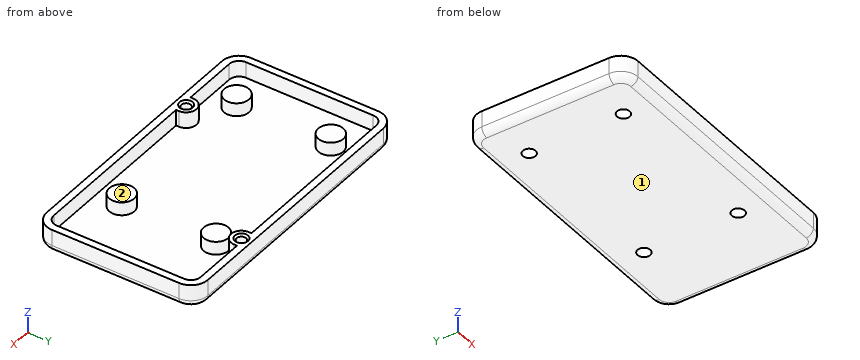
from build123d import *

# Parameters (mm, degrees)
PAD_DEPTH         = 3.4
THICKNESS_T       = 1.5
CYLINDER_W        = 2.2
CYLINDER_H        = 3.4
CYLINDER_ANGLE    = 180
BOX004_W          = 4.4
BOX004_H          = 0.6
BOX004_DEPTH      = 3.4
CYLINDER002_R     = 1
CYLINDER002_DEPTH = 3.9
CHAMFER_SIZE      = 0.4
CYLINDER003_W     = 2.2
CYLINDER003_H     = 3.4
CYLINDER003_ANGLE = 180
BOX006_W          = 4.4
BOX006_H          = 0.6
BOX006_DEPTH      = 3.4
CYLINDER004_R     = 1
CYLINDER004_DEPTH = 3.9
CHAMFER001_SIZE   = 0.4
SKETCH004_R       = 2.65
PAD002_DEPTH      = 2.8
SKETCH005_R       = 1.35
POCKET001_DEPTH   = 3.5


with BuildPart() as part:
    # Sketch → Pad (new body)
    with BuildSketch(Plane.XY):
        with BuildLine():
            Line((2, 31.1), (55.5, 31.1))
            ThreePointArc((57.6, 29), (56.984924, 30.484924), (55.5, 31.1))
            Line((57.6, 29), (57.6, 2))
            ThreePointArc((55.5, -0.1), (56.984924, 0.515076), (57.6, 2))
            Line((55.5, -0.1), (2, -0.1))
            ThreePointArc((-0.1, 2), (0.515076, 0.515076), (2, -0.1))
            Line((-0.1, 2), (-0.1, 29))
            ThreePointArc((2, 31.1), (0.515076, 30.484924), (-0.1, 29))
        make_face()
    extrude(amount=-PAD_DEPTH)

    # Thickness
    thickness_openings = [part.faces().sort_by_distance(p)[0] for p in [
        (28.75, 15.5, 0),
    ]]
    offset(amount=THICKNESS_T, openings=thickness_openings)

    # Cylinder → Cylinder (revolve)
    with BuildSketch(Plane(origin=(16, 0.5, -3.4), x_dir=(1, 0, 0), z_dir=(0, -1, 0))):
        with Locations((1.1, 1.7)):
            Rectangle(CYLINDER_W, CYLINDER_H)
    revolve(axis=Axis((16, 0.5, -3.4), (0, 0, 1)), revolution_arc=CYLINDER_ANGLE)

    # Box004 → Box004 (join)
    with BuildSketch(Plane(origin=(13.8, -0.1, -3.4), x_dir=(1, 0, 0), z_dir=(0, 0, 1))):
        with Locations((2.2, 0.3)):
            Rectangle(BOX004_W, BOX004_H)
    extrude(amount=BOX004_DEPTH)

    # Cylinder002 → Cylinder002 (cut)
    with BuildSketch(Plane(origin=(16, 0.5, -3.9), x_dir=(1, 0, 0), z_dir=(0, 0, 1))):
        Circle(CYLINDER002_R)
    extrude(amount=CYLINDER002_DEPTH, mode=Mode.SUBTRACT)

    # Chamfer
    chamfer_edges = [part.edges().sort_by_distance(p)[0] for p in [
        (16, 1.5, 0),
        (16, -0.5, 0),
        (15.051317, 0.183772, 0),
        (16.948683, 0.183772, 0),
    ]]
    chamfer(chamfer_edges, length=CHAMFER_SIZE)

    # Cylinder003 → Cylinder003 (revolve)
    with BuildSketch(Plane(origin=(42.25, 30.5, -3.4), x_dir=(-1, 0, 0), z_dir=(0, 1, 0))):
        with Locations((1.1, 1.7)):
            Rectangle(CYLINDER003_W, CYLINDER003_H)
    revolve(axis=Axis((42.25, 30.5, -3.4), (0, 0, 1)), revolution_arc=CYLINDER003_ANGLE)

    # Box006 → Box006 (join)
    with BuildSketch(Plane(origin=(40.05, 30.5, -3.4), x_dir=(1, 0, 0), z_dir=(0, 0, 1))):
        with Locations((2.2, 0.3)):
            Rectangle(BOX006_W, BOX006_H)
    extrude(amount=BOX006_DEPTH)

    # Cylinder004 → Cylinder004 (cut)
    with BuildSketch(Plane(origin=(42.25, 30.5, -3.9), x_dir=(1, 0, 0), z_dir=(0, 0, 1))):
        Circle(CYLINDER004_R)
    extrude(amount=CYLINDER004_DEPTH, mode=Mode.SUBTRACT)

    # Chamfer001
    chamfer001_edges = [part.edges().sort_by_distance(p)[0] for p in [
        (42.25, 31.5, 0),
        (43.198683, 30.816228, 0),
        (42.25, 29.5, 0),
        (41.301317, 30.816228, 0),
    ]]
    chamfer(chamfer001_edges, length=CHAMFER001_SIZE)

    # Sketch004 → Pad002 (join)
    with BuildSketch(Plane.XY.offset(-3.4)):
        with Locations((7.8, 5.5)):
            Circle(SKETCH004_R)
        with Locations((42.8, 5.5)):
            Circle(SKETCH004_R)
        with Locations((7.8, 25.5)):
            Circle(SKETCH004_R)
        with Locations((42.8, 25.5)):
            Circle(SKETCH004_R)
    extrude(amount=PAD002_DEPTH)

    # Sketch005 → Pocket001 (cut)
    with BuildSketch(Plane.XY.offset(-4.9)):
        with Locations((7.8, 5.5)):
            Circle(SKETCH005_R)
        with Locations((42.8, 5.5)):
            Circle(SKETCH005_R)
        with Locations((7.8, 25.5)):
            Circle(SKETCH005_R)
        with Locations((42.8, 25.5)):
            Circle(SKETCH005_R)
    extrude(amount=POCKET001_DEPTH, mode=Mode.SUBTRACT)


solid = part.part
Part model, mm, in its own coordinate system. Face numbers are marked on the shaded views. Round coordinates to 2 decimals unless told otherwise and drop trailing zeros. Write each loop counter-clockwise with the first axis right and the second up, starting at its lowest first coordinate (ties: lowest second). Pieces come first, ordered by that corner, then holes. Notation, with made-up numbers: M 63,-3.5 L 88,-3.5 A11 cw 88,15.5 Z; hole C -20.75,8 d11. An arc over 180 degrees is marked long. Return JSON: item names as keys, results as strings. Group by question number.
(1) Saw through at B-B on x = 7.8. Write the cut outline in (y, z).
(2) Saw through at C-C on y = 5.5. Write the cut outline in (x, z).
(3) Two-plate mould, pull along Y, no slides. Class the marked faces 1 and 2: +Y half, -Y half, draft (parallel to the pull), parting line (faces both ways), or undercut.
(4) Saw through at D-D on x = 20.5. Write the cut outline in (y, z), then the cut area to 3 significant figures.
(5) Pin check, flat tips, straight feed: pin 1 Ø2 at (x, y) = (43, 25.5) entering from -Z; pin 2 Ø4.5 at (x, y) = (42.8, 25.5) entering from +Z; pin 3 Ø0.7 at (y, z) = (0, -2) entering from +X. Stop position of each tip, or through.
(6) Drill centre lines: probe 1 along Y at (x, z) = (55.5, -0.65); probe 2 along Y at (x, z) = (16, -2.95); probe 3 along Y at (x, z) = (42, -4.5). Where is each one in solid material? Low to high.
(7) Saw through at A-A on y = 19. Write the cut outline in (x, z), then the cut area to 3 significant figures.
Returned:
{
 "1": {"outline": "M -1.6,-3.4 A1.5 ccw -0.1,-4.9 L 4.15,-4.9 L 4.15,-1.4 L 6.85,-1.4 L 6.85,-4.9 L 24.15,-4.9 L 24.15,-1.4 L 26.85,-1.4 L 26.85,-4.9 L 31.1,-4.9 A1.5 ccw 32.6,-3.4 L 32.6,0 L 31.1,0 L 31.1,-3.4 L 28.15,-3.4 L 28.15,-0.6 L 22.85,-0.6 L 22.85,-3.4 L 8.15,-3.4 L 8.15,-0.6 L 2.85,-0.6 L 2.85,-3.4 L -0.1,-3.4 L -0.1,0 L -1.6,0 Z"},
 "2": {"outline": "M -1.6,-3.4 A1.5 ccw -0.1,-4.9 L 6.45,-4.9 L 6.45,-1.4 L 9.15,-1.4 L 9.15,-4.9 L 41.45,-4.9 L 41.45,-1.4 L 44.15,-1.4 L 44.15,-4.9 L 57.6,-4.9 A1.5 ccw 59.1,-3.4 L 59.1,0 L 57.6,0 L 57.6,-3.4 L 45.45,-3.4 L 45.45,-0.6 L 40.15,-0.6 L 40.15,-3.4 L 10.45,-3.4 L 10.45,-0.6 L 5.15,-0.6 L 5.15,-3.4 L -0.1,-3.4 L -0.1,0 L -1.6,0 Z"},
 "3": {"face 1": "draft", "face 2": "undercut"},
 "4": {"outline": "M -1.6,-3.4 A1.5 ccw -0.1,-4.9 L 31.1,-4.9 A1.5 ccw 32.6,-3.4 L 32.6,0 L 31.1,0 L 31.1,-3.4 L -0.1,-3.4 L -0.1,0 L -1.6,0 Z", "area": "60.5 mm²"},
 "5": {"pin 1": "z = -1.4", "pin 2": "z = -0.6", "pin 3": "x = 58.7"},
 "6": {"probe 1": "-1.6 to -0.1, 31.1 to 32.6", "probe 2": "-1.6 to -0.5, 1.5 to 2.7, 31.1 to 32.6", "probe 3": "-1.12 to 4.41, 6.59 to 24.41, 26.59 to 32.12"},
 "7": {"outline": "M -1.6,-3.4 A1.5 ccw -0.1,-4.9 L 57.6,-4.9 A1.5 ccw 59.1,-3.4 L 59.1,0 L 57.6,0 L 57.6,-3.4 L -0.1,-3.4 L -0.1,0 L -1.6,0 Z", "area": "100 mm²"}
}
